Build history of the part. All positions in model axes, mm. Face numbers are marked on the shaded views. A direction names the side the tool comes from. Coordinates: 2 decimals unless noted, no trailing zeros. Order: outer loops, then holes, each group sorted by start corner. A loop starts at its lowest first (then second) coordinate and runs counter-clockwise, first axis right, second up. Notation, with made-up numbers: M 8.5,29 L 24.5,29 A13 cw 24.5,51 Z; hole C 80,2.5 d3. An arc over 180 degrees is marked long. Write item = value, one per line. Start each with the question number.
Q1. Pin check, flat tips, straight feed: P1, Ø1, axis at x = -4.5, z = -2.5, coming from the +Y side; P2, Ø6, axis at y = 16.5, z = 2.5, coming from the +X side; P3, Ø3, axis at x = 0.5, y = 35, coming from the -Z side; P4, Ø2, axis at y = 36.5, z = -4.5, coming from the -X side. Stop position of each tip, or through.
Q2. Band-saw the part on A-A on z = 1.75. Write the cut outline in (x, y).
Q3. Band-saw the part on D-D on z = -5. Write the cut outline in (x, y).
Q4. Band-saw the part on B-B on y = 34. Write the cut outline in (x, z), plus the area to 3 significant figures.
Q5. Drill centre lines: probe 1 along Y at (x, z) = (3.25, -2); probe 2 along Z at (x, y) = (3, 31.5); probe 3 along Y at (x, z) = (-3.5, -3.25). Where is each one in solid material? Low to high.
Q6. 3-axis set-ups, long thin cutter, end or side, ignore diameter. For the marked faces 1, 2, 3, 4 and 5: which of +Z, -Z, +X, -X, +Y, -Y reach the whole face in a straight line?
Q7. Band-saw the part on C-C on x = -1. Write the cut outline in (y, z).
```python
from build123d import *

# Parameters (mm, degrees)
SKETCH2_W           = 6
SKETCH2_H           = 6
BOSS_EXTRUDE1_DEPTH = 6


with BuildPart() as part:
    # Sketch1 → Revolve1 (revolve)
    with BuildSketch(Plane(origin=(0, 0, 0), x_dir=(0, 0, -1), z_dir=(1, 0, 0))):
        Polygon((0, 46.5), (3, 46.5), (3, 32.5), (4, 32.5), (4, -1.5), (6, -1.5), (6, -4.5), (4, -4.5), (4, -46.5), (0, -46.5), align=None)
    revolve(axis=Axis((0, 46.5, 0), (0, -1, 0)))

    # Sketch2 → Boss-Extrude1 (add)
    with BuildSketch(Plane(origin=(0, 32.5, 0), x_dir=(1, 0, 0), z_dir=(0, 1, 0))):
        Rectangle(SKETCH2_W, SKETCH2_H)
    extrude(amount=BOSS_EXTRUDE1_DEPTH)


solid = part.part
```
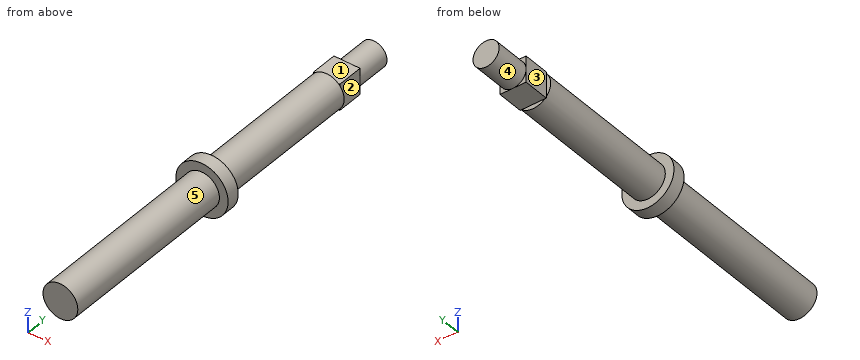
Recorded:
q1.P1 = -1.5
q1.P2 = 4
q1.P3 = -3
q1.P4 = through
q2.outline = M -5.74,-4.5 L -3.6,-4.5 L -3.6,-46.5 L 3.6,-46.5 L 3.6,-4.5 L 5.74,-4.5 L 5.74,-1.5 L 3.6,-1.5 L 3.6,32.5 L 3,32.5 L 3,38.5 L 2.44,38.5 L 2.44,46.5 L -2.44,46.5 L -2.44,38.5 L -3,38.5 L -3,32.5 L -3.6,32.5 L -3.6,-1.5 L -5.74,-1.5 Z
q3.outline = M -3.32,-4.5 L 3.32,-4.5 L 3.32,-1.5 L -3.32,-1.5 Z
q4.outline = M -3,-3 L 3,-3 L 3,3 L -3,3 Z
q4.area = 36.0 mm2
q5.probe_1 = -46.5 to 32.5
q5.probe_2 = -2.65 to 2.65
q5.probe_3 = -4.5 to -1.5
q6.face_1 = +Z, +X, -X, +Y
q6.face_2 = +Z, -Z, +X, +Y
q6.face_3 = +Z, -Z, -X, +Y
q6.face_4 = +Y
q6.face_5 = -Y
q7.outline = M -46.5,-3.87 L -4.5,-3.87 L -4.5,-5.92 L -1.5,-5.92 L -1.5,-3.87 L 32.5,-3.87 L 32.5,-3 L 38.5,-3 L 38.5,-2.83 L 46.5,-2.83 L 46.5,2.83 L 38.5,2.83 L 38.5,3 L 32.5,3 L 32.5,3.87 L -1.5,3.87 L -1.5,5.92 L -4.5,5.92 L -4.5,3.87 L -46.5,3.87 Z
